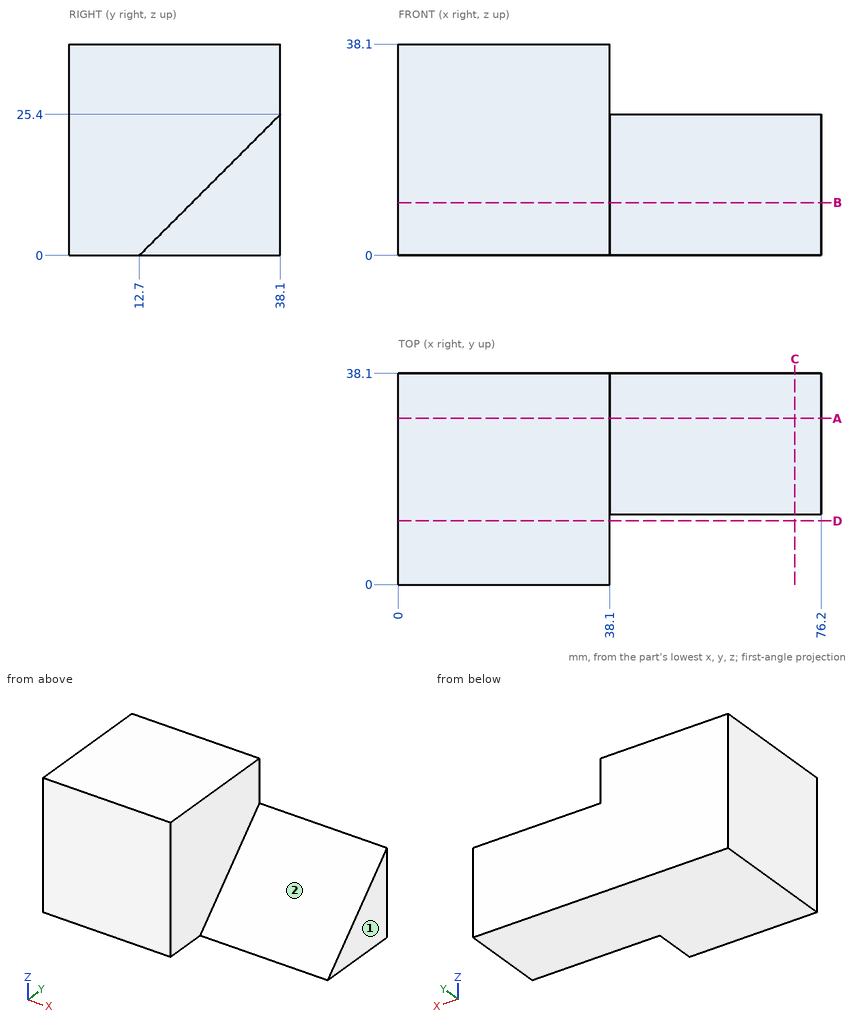
Design review of the part shown in the three views and the two pictorial views. Dimensions are in mm from the part's minimum x, y and z. A direction names the side the tool comes from. Round coordinates to 2 decimals unless told otherwise and drop trailing zeros. Loops run counter-clockwise (first coordinate to the right, second up) from the corner with the lowest first, then second, coordinate; pieces in that order, holes last.
Q1. Add section D-D on y = 11.5. Write out the cut boundary in (x, z).
Result sheet:
outline: (0, 0) - (38.1, 0) - (38.1, 38.1) - (0, 38.1) - close
Q2. Add section C-C on x = 71.5. Write out the cut boundary in (y, z).
Result sheet:
outline: (12.7, 0) - (38.1, 0) - (38.1, 25.4) - close
Q3. Insertion check: pin 1 Ø8 at (x, y) = (62, 6.5) entering from -Z (3 decimals); pin 2 Ø11.5 at (y, z) = (13.5, 27.5) entering from +X; pin 3 Ø4 at (x, z) = (54, 12.5) entering from -Y; pin 4 Ø5 at (x, y) = (57.5, 34.5) entering from +Z. Each pin has a flat end and moves straight along its axis. Give the tip position at first contact, or say it passes through.
Result sheet:
pin 1: passes through
pin 2: stops at x = 38.1
pin 3: stops at y = 23.2
pin 4: stops at z = 24.3
Q4. Add section A-A on y = 30. Write out the cut boundary in (x, z).
Result sheet:
outline: (0, 0) - (76.2, 0) - (76.2, 17.3) - (38.1, 17.3) - (38.1, 38.1) - (0, 38.1) - close
Q5. Add section B-B on z = 9.5. Write out the cut boundary in (x, y), plus the area to 3 significant figures.
Result sheet:
outline: (0, 0) - (38.1, 0) - (38.1, 22.2) - (76.2, 22.2) - (76.2, 38.1) - (0, 38.1) - close
area: 2,060 mm2
Q6. To check wall thickness, follow line 1 along X through (y, z) = (5.5, 22); line 2 along Z through (x, y) = (50.5, 33); line 3 along Y through (x, z) = (60, 3.5). State the ranges of each line that lie inside material, in increasing order.
Result sheet:
line 1: x = 0 to 38.1
line 2: z = 0 to 20.3
line 3: y = 16.2 to 38.1
Q7. Machinability: for the marked faces 1 and 2, which of the approach directions +Z, -Z, +X, -X, +Y, -Y give a long, thin tool a straight path to every point of the face, cutting with its end or side? Answer none if there is none.
Result sheet:
face 1: +Z, -Z, +X, +Y, -Y
face 2: +Z, +X, -Y
